Could you check a few things on this model? Use its own coordinates, in mm. A direction names the side the tool comes from. Round coordinates to 2 decimals unless told otherwise and drop trailing zeros. Loops run counter-clockwise (first coordinate to the right, second up) from the corner with the lowest first, then second, coordinate; pieces in that order, holes last. Notation, with made-up numbers: M -4.75,32.5 L 54.25,32.5 A25 cw 54.25,59.5 Z; hole C 72,25.25 d6. An arc over 180 degrees is marked long. Return JSON: item names as keys, results as strings. Group by question number.
```python
from build123d import *

# Parameters (mm, degrees)
F0_W     = 45
F0_H     = 90
F1_DEPTH = 1400
F3_DEPTH = 1110.001
F5_DEPTH = 45.001
F6_W     = 1200
F6_H     = 600
F7_DEPTH = 8


with BuildPart() as f1:
    # F0 (on Top) → F1 (new body)
    with BuildSketch(Plane.XY):
        with Locations((-532.5, 45)):
            Rectangle(F0_W, F0_H)
    extrude(amount=F1_DEPTH)


with BuildPart() as f1b:
    # F0 (on Top) → F1, piece 2 (new body)
    with BuildSketch(Plane.XY):
        with Locations((532.5, 45)):
            Rectangle(F0_W, F0_H)
    extrude(amount=F1_DEPTH)


with BuildPart() as f3_tool:
    # F2 (on face) → F3 (new body, through all)
    with BuildSketch(Plane(origin=(-555, 0, 0), x_dir=(0, -1, 0), z_dir=(-1, 0, 0))):
        Polygon((0, 1400), (-90, 1400), (-90, 1370), align=None)
    extrude(amount=-F3_DEPTH)


with BuildPart() as f1_1:
    add(f1.part)

    # F3: cut by f3_tool
    add(f3_tool.part, mode=Mode.SUBTRACT)

    # F4 (on face) → F5 (cut, through all)
    with BuildSketch(Plane(origin=(510, 0, 0), x_dir=(0, -1, 0), z_dir=(-1, 0, 0))):
        Polygon((0, 1400), (-90, 1400), (-90, 1370), align=None)
    extrude(amount=-F5_DEPTH, mode=Mode.SUBTRACT)



with BuildPart() as f1b_1:
    add(f1b.part)

    # F3: cut by f3_tool
    add(f3_tool.part, mode=Mode.SUBTRACT)


with BuildPart() as f1_2:
    add(f1_1.part)

    add(f1b_1.part)  # F7 merges F1b
    # F6 (on face) → F7 (join)
    with BuildSketch(Plane(origin=(0, 420, 1260), x_dir=(1, 0, 0), z_dir=(0, 0.316227766, 0.9486832981))):
        with Locations((0, -297.8505426185)):
            Rectangle(F6_W, F6_H)
    extrude(amount=F7_DEPTH)


solid = f1_2.part
```
1. I need wall thicknesses on probe 1 along X at (y, z) = (15, 626.5); probe 2 along Z at (x, y) = (198, 67.5); probe 3 along Y at (x, z) = (-542.5, 1231.5). Which ranges of each line are inside material? Lowest first, please.
2. We'd pull the mould along X, two halves only. Please class faces 3 (the face through (-555, 44, 690)), 4 (the face through (-533, 0, 690)), 5 (the face through (-510, 44, 690)): +X half, -X half, draft (parallel to the pull), parting line (faces both ways), or undercut.
3. If we section it at A-A, the plane z = 754: Please give me the cut outline in (x, y), then the cut area to 3 significant figures.
4. I'm going to push flat-ended pins straight in: pin 1 Ø3 at (x, y) = (-403.5, 364) entering from -Z; pin 2 Ø8 at (x, y) = (-77.5, 37.5) entering from -Z; pin 3 Ø1.5 at (x, y) = (-312.5, 226.5) entering from -Z. Where does each tip first touch, or does it pass through?
5. If we section it at B-B, the plane y = 18: Please give me the cut outline in (x, z).
6. If we section it at D-D, the plane y = 259.5: Please give me the cut outline in (x, z), then the cut area to 3 significant figures.
7. On a 3-axis mill with a long thin cutter (end or side, diameter ignored), from which of +Z, -Z, +X, -X, +Y, -Y can I reach the whole of each face in a straight line? I mean faces 1 (the face through (-600, 135, 1359)), 2 (the face through (532, 0, 690)). Say none if no direction works.
8. If we section it at C-C, the plane x = 330: Please give me the cut outline in (y, z).
Geometry results:
{
 "1": {"probe 1": "-555 to -510, 510 to 555", "probe 2": "1377.5 to 1385.93", "probe 3": "0 to 90"},
 "2": {"face 3": "-X half", "face 4": "draft", "face 5": "undercut"},
 "3": {"outline": "M -555,0 L -510,0 L -510,90 L -555,90 Z; M 510,0 L 555,0 L 555,90 L 510,90 Z", "area": "8,100 mm^2"},
 "4": {"pin 1": "z = 1278.17", "pin 2": "z = 1386.17", "pin 3": "z = 1324.25"},
 "5": {"outline": "M -600,1394 L -555,1394 L -555,0 L -510,0 L -510,1394 L 510,1394 L 510,0 L 555,0 L 555,1394 L 600,1394 L 600,1402.43 L -600,1402.43 Z"},
 "6": {"outline": "M -600,1313.5 L 600,1313.5 L 600,1321.93 L -600,1321.93 Z", "area": "10,100 mm^2"},
 "7": {"face 1": "+Z, -Z, -X, +Y, -Y", "face 2": "-Z, +X, -X, -Y"},
 "8": {"outline": "M -147.17,1449.06 L 422.04,1259.32 L 424.57,1266.91 L -144.64,1456.65 Z"}
}
